For this review, take the finished solid that the model builds, in its own axes (mm). Face numbers are marked on the shaded views. Coordinates: 2 decimals unless noted, no trailing zeros. Order: outer loops, then holes, each group sorted by start corner. A loop starts at its lowest first (then second) coordinate and runs counter-clockwise, first axis right, second up.
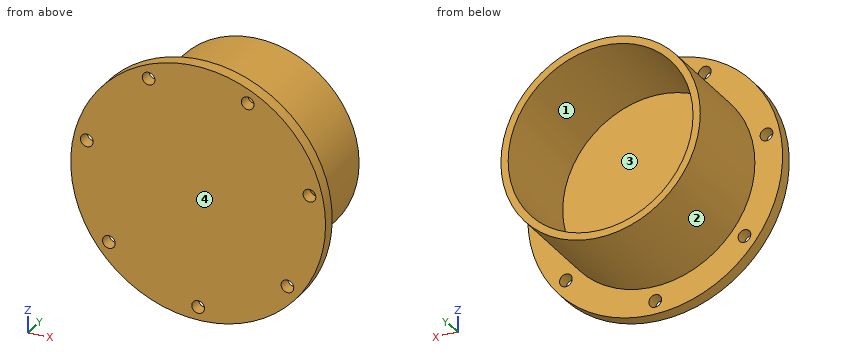
from build123d import *

# Parameters (mm, degrees)
SKETCH2_R           = 35.15
SKETCH2_R_2         = 1.75
BOSS_EXTRUDE1_DEPTH = 3.5
SKETCH3_R           = 27.5
SKETCH3_R_2         = 25.5
BOSS_EXTRUDE2_DEPTH = 28.7


with BuildPart() as part:
    # Sketch2 → Boss-Extrude1 (new body)
    with BuildSketch(Plane(origin=(0, 0, 0), x_dir=(1, 0, 0), z_dir=(0, 1, 0))):
        Circle(SKETCH2_R)
        with Locations((0, 31.5)):
            Circle(SKETCH2_R_2, mode=Mode.SUBTRACT)
        with Locations((24.627691698, 19.639928759)):
            Circle(SKETCH2_R_2, mode=Mode.SUBTRACT)
        with Locations((30.710229234, -7.00940942)):
            Circle(SKETCH2_R_2, mode=Mode.SUBTRACT)
        with Locations((13.667337782, -28.380519339)):
            Circle(SKETCH2_R_2, mode=Mode.SUBTRACT)
        with Locations((-13.667337782, -28.380519339)):
            Circle(SKETCH2_R_2, mode=Mode.SUBTRACT)
        with Locations((-30.710229234, -7.00940942)):
            Circle(SKETCH2_R_2, mode=Mode.SUBTRACT)
        with Locations((-24.627691698, 19.639928759)):
            Circle(SKETCH2_R_2, mode=Mode.SUBTRACT)
    extrude(amount=BOSS_EXTRUDE1_DEPTH)

    # Sketch3 → Boss-Extrude2 (add)
    with BuildSketch(Plane(origin=(0, 3.5, 0), x_dir=(1, 0, 0), z_dir=(0, 1, 0))):
        Circle(SKETCH3_R)
        Circle(SKETCH3_R_2, mode=Mode.SUBTRACT)
    extrude(amount=BOSS_EXTRUDE2_DEPTH)


solid = part.part
1. Take a section at C-C, the plane z = -31.5. Give the boundary of the cut face in (x, y), plus the area to 3 significant figures.
Answer below:
outline: (-15.6, 0) - (-1.75, 0) - (-1.75, 3.5) - (-15.6, 3.5) - close; (1.75, 0) - (15.6, 0) - (15.6, 3.5) - (1.75, 3.5) - close
area: 96.9 mm2
2. Take a section at D-D, the plane z = 0. Give the boundary of the cut face in (x, y), plus the area to 3 significant figures.
Answer below:
outline: (-35.15, 0) - (35.15, 0) - (35.15, 3.5) - (27.5, 3.5) - (27.5, 32.2) - (25.5, 32.2) - (25.5, 3.5) - (-25.5, 3.5) - (-25.5, 32.2) - (-27.5, 32.2) - (-27.5, 3.5) - (-35.15, 3.5) - close
area: 361 mm2
3. Clearance check with flat-ended pins moving along their axes: pin 1 Ø12 at (x, y) = (21.5, 27.5) entering from -Z; pin 2 Ø4 at (x, z) = (-13.67, 28.38) entering from +Y; pin 3 Ø8 at (y, z) = (6.5, 19.5) entering from -X. State where each tip first meets the part, or that it passes through.
Answer below:
pin 1: stops at z = -22.72
pin 2: stops at y = 3.5
pin 3: stops at x = -30.85
4. The part is to be moulded in two halves that separate along Z. For the marked faces 1, 2, 3 and 4, say which applies: +Z half, -Z half, draft (parallel to the pull), parting line (faces both ways), or undercut.
Answer below:
face 1: undercut
face 2: parting line
face 3: undercut
face 4: draft
5. Take a section at B-B, the plane y = 2. Give the boundary of the cut face in (x, z).
Answer below:
outline: circle Ø70.3 at (0, 0); hole circle Ø3.5 at (-30.71, 7.01); hole circle Ø3.5 at (-24.63, -19.64); hole circle Ø3.5 at (-13.67, 28.38); hole circle Ø3.5 at (0, -31.5); hole circle Ø3.5 at (13.67, 28.38); hole circle Ø3.5 at (24.63, -19.64); hole circle Ø3.5 at (30.71, 7.01)
6. Take a section at A-A, the plane x = 0. Give the boundary of the cut face in (y, z), plus the area to 3 significant figures.
Answer below:
outline: (0, -35.15) - (3.5, -35.15) - (3.5, -33.25) - (0, -33.25) - close; (0, -29.75) - (3.5, -29.75) - (3.5, -27.5) - (32.2, -27.5) - (32.2, -25.5) - (3.5, -25.5) - (3.5, 25.5) - (32.2, 25.5) - (32.2, 27.5) - (3.5, 27.5) - (3.5, 35.15) - (0, 35.15) - close
area: 349 mm2
7. To check wall thickness, follow L1, parallel to Z at x = 0, y = 2; L2, parallel to Z at x = -0.5, y = 11. State the ranges of each line that lie inside material, in increasing order.
Answer below:
L1: z = -35.15 to -33.25, -29.75 to 35.15
L2: z = -27.5 to -25.5, 25.5 to 27.5
